from build123d import *

# Parameters (mm, degrees)
BOX004_W       = 52
BOX004_H       = 15
BOX004_DEPTH   = 3.25
BOX003_W       = 56.3
BOX003_H       = 19.4
BOX003_DEPTH   = 3.25
BOX005_W       = 52
BOX005_H       = 15
BOX005_DEPTH   = 3.25
CYLINDER_R     = 0.35
CYLINDER_DEPTH = 0.4
ARRAY_X_COUNT  = 16
ARRAY_X_PITCH  = 1.27
BOX_W          = 59
BOX_H          = 29.3
BOX_DEPTH      = 0.4
BOX002_W       = 56.3
BOX002_H       = 19.4
BOX002_DEPTH   = 3.25
BOX001_W       = 59
BOX001_H       = 26
BOX001_DEPTH   = 3.25


with BuildPart() as box004:
    # Box004 → Box004 (new body)
    with BuildSketch(Plane(origin=(3.5, 6.3, 0.4), x_dir=(1, 0, 0), z_dir=(0, 0, 1))):
        with Locations((26, 7.5)):
            Rectangle(BOX004_W, BOX004_H)
    extrude(amount=BOX004_DEPTH)


with BuildPart() as cut001:
    # Box003 → Box003 (new body)
    with BuildSketch(Plane(origin=(1.35, 4.1, 0.4), x_dir=(1, 0, 0), z_dir=(0, 0, 1))):
        with Locations((28.15, 9.7)):
            Rectangle(BOX003_W, BOX003_H)
    extrude(amount=BOX003_DEPTH)

    # Cut001: cut Box004
    add(box004.part, mode=Mode.SUBTRACT)


with BuildPart() as box005:
    # Box005 → Box005 (new body)
    with BuildSketch(Plane(origin=(3.5, 6.3, 0.4), x_dir=(1, 0, 0), z_dir=(0, 0, 1))):
        with Locations((26, 7.5)):
            Rectangle(BOX005_W, BOX005_H)
    extrude(amount=BOX005_DEPTH)


with BuildPart() as array:
    # Cylinder → Cylinder (new body)
    with BuildSketch(Plane(origin=(21.5, 27.8, 0), x_dir=(1, 0, 0), z_dir=(0, 0, 1))):
        Circle(CYLINDER_R)
    extrude(amount=CYLINDER_DEPTH)

    # Array X: Array ×16


with BuildPart() as array_1:
    add(array.part)
    with Locations(*[(i * ARRAY_X_PITCH, 0, 0) for i in range(1, ARRAY_X_COUNT)]):
        add(array.part)


with BuildPart() as cut002:
    # Box → Box (new body)
    with BuildSketch(Plane.XY):
        with Locations((29.5, 14.65)):
            Rectangle(BOX_W, BOX_H)
    extrude(amount=BOX_DEPTH)

    # Cut002: cut Array
    add(array_1.part, mode=Mode.SUBTRACT)


with BuildPart() as box002:
    # Box002 → Box002 (new body)
    with BuildSketch(Plane(origin=(1.35, 4.1, 0.4), x_dir=(1, 0, 0), z_dir=(0, 0, 1))):
        with Locations((28.15, 9.7)):
            Rectangle(BOX002_W, BOX002_H)
    extrude(amount=BOX002_DEPTH)


with BuildPart() as fusion:
    # Box001 → Box001 (new body)
    with BuildSketch(Plane.XY.offset(0.4)):
        with Locations((29.5, 13)):
            Rectangle(BOX001_W, BOX001_H)
    extrude(amount=BOX001_DEPTH)

    # Cut: cut Box002
    add(box002.part, mode=Mode.SUBTRACT)

    # Fusion: union Cut001, box005, Cut002
    add(cut001.part)
    add(box005.part)
    add(cut002.part)


solid = fusion.part
Design review of the part built by this model. Coordinates are the model's own, in mm. A direction names the side the tool comes from. Round coordinates to 2 decimals unless told otherwise and drop trailing zeros. Loops run counter-clockwise (first coordinate to the right, second up) from the corner with the lowest first, then second, coordinate; pieces in that order, holes last. Notation, with made-up numbers: M 22,77.5 L 52,77.5 A18 cw 52,106.5 Z; hole C -37,46.25 d1. An arc over 180 degrees is marked long. Answer as a JSON object with one key per item and string values.
Item 1: We need section A-A on x = 10. Give the boundary of the cut face in (y, z), and give its area (3 significant figures).
Answer sheet:
{"outline": "M 0,0 L 29.3,0 L 29.3,0.4 L 26,0.4 L 26,3.65 L 0,3.65 Z", "area": "96.2 mm^2"}
Item 2: Machinability: for faces 1 (the flat face through (29, 13, 3.65)), 2 (the flat face through (29, 27, 0.4)), which of the approach directions +Z, -Z, +X, -X, +Y, -Y give a long, thin tool a straight path to every point of the face, cutting with its end or side? Answer none if there is none.
Answer sheet:
{"face 1": "+Z, +X, -X, +Y, -Y", "face 2": "+Z, +X, -X, +Y"}
Item 3: Clearance check with flat-ended pins moving along their axes: P1, Ø3.5, axis at x = 44, y = 28, coming from the +Z side; P2, Ø1.6, axis at x = 29.5, z = 1.5, coming from the +Y side. State where each tip first meets the part, or that it passes through.
Answer sheet:
{"P1": "stops at z = 0.4", "P2": "stops at y = 26"}
Item 4: We need section B-B on z = 2.3. Give the boundary of the cut face in (x, y), and give its area (3 significant figures).
Answer sheet:
{"outline": "M 0,0 L 59,0 L 59,26 L 0,26 Z", "area": "1,530 mm^2"}
Item 5: Wall thickness on L1, parallel to Y at x = 29.12, z = 0.25; L2, parallel to Y at x = 4, z = 0.85: over which ranges is each line inside the solid? List them lowest first. Write a range as from..to.
Answer sheet:
{"L1": "y = 0..27.45, 28.15..29.3", "L2": "y = 0..26"}
